Verification items for the finished model (mm, model axes). A direction names the side the tool comes from. Coordinates: 2 decimals unless noted, no trailing zeros. Order: outer loops, then holes, each group sorted by start corner. A loop starts at its lowest first (then second) coordinate and runs counter-clockwise, first axis right, second up. Notation, with made-up numbers: M 14.5,18 L 73.5,18 A27 ccw 73.5,56 Z; hole C 16.25,82.5 d5. An arc over 180 degrees is marked long. Answer as a JSON object with one key per item and string values. Group by question number.
(1) Cross-section at B-B (x = -40). Enter the section's corners in (y, z).
(2) Access from +Z, -Z, +X, -X, +Y, -Y to the whole of each face (thin tool, end or side, straight path). Record for faces 5 (the face through (-52.697, -4.056, -9.736)), 6 (the face through (7.203, -6.859, 4.084)), 7 (the face through (18.4, -5.2, 15.1)), 8 (the face through (-1, 0, -13)), 9 (the face through (-1.93, -1.141, -6.203)).
(3) Gauge pin test, flat end, axial feed: pin 1 Ø3 at (x, y) = (20, -4) entering from +Z. Record the tip position at first contact, or that the pin passes through.
(4) Cross-section at A-A (z = 0). Count the separate pieces of the cut face and the enclosed holes in it, plus the area to 3 significant figures.
(5) Cross-section at C-C (z = -13). Enter the section's corners in (x, y), plus the area to 3 significant figures.
(6) Material ranges on line 1 (Y direction, x = 60, z = 16); line 2 (Z direction, x = -40, y = -4); line 3 (Z direction, x = 27.5, y = -4), recorded low to high.
(7) Mould release check, pull along Z, two halves, no side actions. Record for faces 1 (the face through (-1, -4, -20)), 2 (the face through (7.203, -1.141, 4.084)), 3 (the face through (24.015, -4.056, 0.703)), 4 (the face through (-60, -4, 10)): released by +Z, released by -Z, zero draft, split by the parting line, or undercut.
(8) Cross-section at D-D (x = -60). Enter the section's corners in (y, z).
from build123d import *

# Parameters (mm, degrees)
F0_W      = 130
F0_H      = 40
F1_DEPTH  = 8
F2_R      = 16
F3_DEPTH  = 8.001
F4_R      = 2
F5_DEPTH  = 10
F7_DEPTH  = 25
F8_R      = 3.99999
F9_R      = 1.5
F10_DEPTH = 25


# Not quite as in the source:
# - a fillet or chamfer is up to 0.001 mm smaller than in the source, because OpenCascade refuses the exact size


with BuildPart() as f1:
    # F0 (on Front) → F1 (new body)
    with BuildSketch(Plane.XZ):
        Rectangle(F0_W, F0_H)
    extrude(amount=F1_DEPTH)

    # F2 (on face) → F3 (cut, through all)
    with BuildSketch(Plane.XZ.offset(8)):
        with Locations((40, 0)):
            Circle(F2_R)
        with Locations((-40, 0)):
            Circle(F2_R)
    extrude(amount=-F3_DEPTH, mode=Mode.SUBTRACT)

    # F4 (on face) → F5 (cut)
    with BuildSketch(Plane.XY.offset(20)):
        with Locations((-60, -4)):
            Circle(F4_R)
        with Locations((60, -4)):
            Circle(F4_R)
        with Locations((-20, -4)):
            Circle(F4_R)
        with Locations((20, -4)):
            Circle(F4_R)
    extrude(amount=-F5_DEPTH, mode=Mode.SUBTRACT)

    # F6 (on face) → F7 (cut)
    with BuildSketch(Plane.XZ.offset(8)):
        with BuildLine():
            Line((3, 13), (-7, 13))
            ThreePointArc((-7, 13), (-9.1213203436, 12.1213203436), (-10, 10))
            Line((-10, 10), (-10, -2))
            ThreePointArc((-10, -2), (-9.1213203436, -4.1213203436), (-7, -5))
            Line((-7, -5), (3, -5))
            ThreePointArc((3, -5), (5.1213203436, -4.1213203436), (6, -2))
            Line((6, -2), (6, 10))
            ThreePointArc((6, 10), (5.1213203436, 12.1213203436), (3, 13))
        make_face()
    extrude(amount=-F7_DEPTH, mode=Mode.SUBTRACT)

    # F8 (radius 4 in the source; OpenCascade refuses exactly that, so slightly less here)
    f8_edges = [f1.edges().sort_by_distance(p)[0] for p in [
        (6, -8, 4),
        (6, 0, 4),
    ]]
    fillet(f8_edges, radius=F8_R)

    # F9 (on face) → F10 (cut)
    with BuildSketch(Plane(origin=(0, 0, 0), x_dir=(-1, 0, 0), z_dir=(0, 1, 0))):
        with Locations((-18, 4)):
            Circle(F9_R)
    extrude(amount=-F10_DEPTH, mode=Mode.SUBTRACT)


solid = f1.part
Taken from the geometry:
{
 "1": {"outline": "M -8,-20 L 0,-20 L 0,-16 L -8,-16 Z; M -8,16 L 0,16 L 0,20 L -8,20 Z"},
 "2": {"face 5": "+Y, -Y", "face 6": "-Y", "face 7": "+Z", "face 8": "+Z, -Z, +X, -X, +Y", "face 9": "+Y"},
 "3": {"pin 1": "stops at z = 10"},
 "4": {"separate pieces": "4", "enclosed holes": "0", "area": "386 mm²"},
 "5": {"outline": "M -65,-8 L -49.33,-8 L -49.33,0 L -65,0 Z; M -30.67,-8 L 30.67,-8 L 30.67,0 L -30.67,0 Z; M 49.33,-8 L 65,-8 L 65,0 L 49.33,0 Z", "area": "742 mm²"},
 "6": {"line 1": "y = -8 to -6, -2 to 0", "line 2": "z = -20 to -16, 16 to 20", "line 3": "z = -20 to -9.99, 9.99 to 20"},
 "7": {"face 1": "released by -Z", "face 2": "undercut", "face 3": "undercut", "face 4": "released by +Z"},
 "8": {"outline": "M -8,-20 L 0,-20 L 0,20 L -2,20 L -2,10 L -6,10 L -6,20 L -8,20 Z"}
}
